Autodesk Fusion 360 part; units mm, degrees
sketch "Main Body" plane through (0, 0, 0) normal (0, 0, 1) x (1, 0, 0)
  circle A0 centre (0, 0) radius 16.85
  line L0 (-20, 20) -> (20, 20)
  line L1 (20, 20) -> (20, -20)
  line L2 (20, -20) -> (-20, -20)
  line L3 (-20, -20) -> (-20, 20)
  line L4 (-20, 15) -> (20, 15)
  point P0 (-20, 0)
  point P1 (0, 20)
  dimension "d1" = 33.7
  dimension "d2" = 40
  dimension "d3" = 15
extrude "Extrude1" add sketch "Main Body" along normal blind 30 contours A0 L1 L2 L3 L4
sketch "Antenna Holder" plane through (20, 0, 0) normal (1, 0, 0) x (0, 1, 0)
  line L0 (-20, 0) -> (15, 0)
  line L1 (15, 0) -> (15, 30)
  line L2 (15, 30) -> (-20, 30)
  line L3 (-20, 30) -> (-20, 0)
  circle A0 centre (-22.2, 9.1) radius 3.2
  line L4 (-23.48, 15) -> (-20, 15)
  line L5 (-20, 15) -> (-20, 0)
  line L6 (-20, 0) -> (-23.48, 0)
  line L7 (-23.48, 0) -> (-23.48, 15)
  point P0 (-23.48, 6.1672)
  dimension "d6" = 6.4
  dimension "d7" = 22.2
  dimension "d8" = 20.9
  dimension "d9" = 1.28
extrude "Extrude2" add sketch "Antenna Holder" against normal blind 40 contours L3 A0 L5 L6 L7 | L3 A0 L5 | L3 A0 L4 L5 L7
extrude "Extrude3" cut sketch "Antenna Holder" against normal blind 40 contours L3 A0 L5
sketch "Coax_Connector_holder" plane through (20, -21.74, 3.3881) normal (1, 0, 0) x (0, 1, 0)
  line L0 (-1.74, 2.779) -> (-13.74, 2.779)
  line L1 (-13.74, 2.779) -> (-13.74, -3.3881)
  line L2 (-13.74, -3.3881) -> (-1.74, -3.3881)
  line L3 (-1.74, -3.3881) -> (-1.74, 2.779)
  line L4 (1.74, -3.3881) -> (36.74, -3.3881)
  line L5 (-1.74, -3.3881) -> (-1.74, 11.6119)
  line L6 (-13.74, -3.3881) -> (-25.74, -3.3881)
  line L7 (-25.74, -3.3881) -> (-25.74, 11.6119)
  line L8 (-25.74, 11.6119) -> (-13.74, 11.6119)
  line L9 (-13.74, 11.6119) -> (-13.74, -3.3881)
  line L10 (-1.74, 11.6119) -> (1.74, 11.6119)
  point P0 (-1.74, 2.779)
  point P1 (-0.46, 5.7119)
  dimension "d15" = 12
  dimension "d16" = 12
extrude "Extrude4" add sketch "Coax_Connector_holder" against normal blind 40
sketch "Connector_Hole" plane through (0, -47.48, 0) normal (0, -1, 0) x (1, 0, 0)
  line L0 (20, 0) -> (20, 15)
  line L1 (20, 15) -> (-20, 15)
  line L2 (-20, 15) -> (-20, 0)
  line L3 (-20, 0) -> (20, 0)
  circle A0 centre (0, 11.1) radius 7.5
  circle A1 centre (0, 11.1) radius 8.5
  line L4 (-20, 30) -> (20, 30)
  line L5 (-20, 14.1) -> (20, 14.1)
  line L6 (-20, 14.5) -> (20, 14.5)
  dimension "d19" = 17
  dimension "d20" = 15
  dimension "d21" = 18.9
  dimension "d22" = 3
  dimension "d23" = 3.4
extrude "Extrude5" cut sketch "Connector_Hole" against normal blind 5.5 contours L0 A1 L5 L6 | L0 L1 A1 L6 | A0 A1 L5 L6 | L2 A1 L5 L6 | L1 A0 A1 L6 | A0 L5 L6 | A0 L5 | L1 L2 A1 L6 | A0 A1 L5 L6 | L1 A0 L6 | L1 A0 A1 L6
extrude "Extrude6" cut sketch "Connector_Hole" against normal blind 15 from surface at -5.5 contours L0 L1 A1 L6 | A0 A1 L5 L6 | A0 A1 L5 | L1 A0 A1 L6 | A0 L5 L6 | A0 L5 | L1 L2 A1 L6 | A0 A1 L5 L6 | L1 A0 L6 | L1 A0 A1 L6
sketch "Sketch5" plane through (0, 0, 15) normal (0, 0, 1) x (-1, 0, 0)
  line L0 (-20, 23.48) -> (-20, 20)
  line L1 (-20, 20) -> (20, 20)
  line L2 (20, 20) -> (20, 23.48)
  line L3 (20, 23.48) -> (-20, 23.48)
  line L4 (12, 20) -> (12, 23.48)
  line L5 (-12, 20) -> (-12, 23.48)
  dimension "d29" = 8
  dimension "d30" = 8
extrude "Extrude7" cut sketch "Sketch5" against normal blind 5 contours L1 L3 L4 L5
equation "d7 = 19 mm + 3.2 mm"
equation "d9 = d6 / 5"
equation "d10 = -d2"
equation "d12 = -d2"
equation "d17 = -d2"
equation "d21 = d8 - 2 mm"
equation "d22 = d20 / 5"
equation "d23 = d19 / 5"
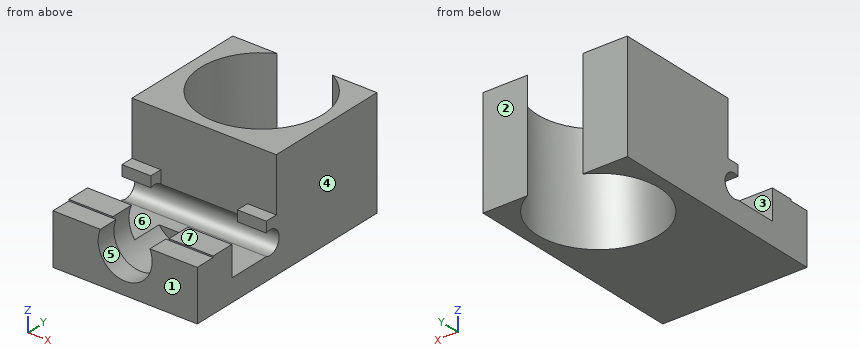
Input: part model. Units: mm. Frame: model coordinates. Face numbers are marked on the shaded views. A direction names the side the tool comes from. Give positions to 0.01 mm unless a question says otherwise; leave off trailing zeros. Order: outer loops, then holes, each group sorted by start corner. A loop starts at its lowest first (then second) coordinate and runs counter-clockwise, first axis right, second up. Notation, with made-up numbers: M 35.5,40 L 82.5,40 A25 cw 82.5,61 Z; hole C -31.5,19 d11. An arc over 180 degrees is marked long. Return JSON: item names as keys, results as strings.
Item 1: Cut plane A-A (y = -22.2). Return loops of the section in (x, z), then the cut area to 3 significant figures.
Solutions:
{"outline": "M -20,0 L 20,0 L 20,5.9 L -20,5.9 Z; M -20,12.3 L -12,12.3 L -12,15 L -20,15 Z; M 12,12.3 L 20,12.3 L 20,15 L 12,15 Z", "area": "279 mm^2"}
Item 2: Ray query, probe 1 along Y at (x, z) = (-9.5, 9); probe 2 along X at (y, z) = (-45.65, 11.1); probe 3 along X at (y, z) = (0, 9). Return the intervals inside material, ascending.
Solutions:
{"probe 1": "-47.48 to -35.48, -19 to -13.92, 13.92 to 15", "probe 2": "-20 to -7.5, 7.5 to 20", "probe 3": "-20 to -16.85, 16.85 to 20"}
Item 3: Pull-direction query (Y, two-part tool) for the marked faces 1, 2, 3 and 4; classes: +Y half, -Y half, draft (parallel to the pull), parting line (faces both ways), or undercut.
Solutions:
{"face 1": "-Y half", "face 2": "+Y half", "face 3": "undercut", "face 4": "draft"}
Item 4: Access query for the marked faces 5, 6 and 7. Directions: +Z, -Z, +X, -X, +Y, -Y. A direction counts if a zero-diameter tool reaches every point of the face in a straight line with its end or side. Return the directions, or none.
Solutions:
{"face 5": "-Y", "face 6": "+Z, +X, -X", "face 7": "+Z, +X, -X, -Y"}
Item 5: First-contact query: P1, Ø5, axis at x = -13.5, y = -37.5, coming from the +Z side; P2, Ø1.6, axis at x = -12.5, y = -43.5, coming from the +Z side; P3, Ø3, axis at x = -1, z = 7.5, coming from the +Y side. Flat tips, straight axial feed; report the tip coordinate or a pass-through.
Solutions:
{"P1": "z = 14.5", "P2": "z = 14.1", "P3": "y = -16.66"}
Item 6: Cut plane B-B (x = -10). Return loops of the section in (y, z).
Solutions:
{"outline": "M -47.48,0 L -13.56,0 L -13.56,30 L -20,30 L -20,11.42 A3.2 cw -23.48,6.17 L -35.48,6.17 L -35.48,14.5 L -41.98,14.5 L -41.98,14.1 L -47.48,14.1 Z; M 13.56,0 L 15,0 L 15,30 L 13.56,30 Z"}
Item 7: Cut plane C-C (z = 9.1). Return loops of the section in (x, y).
Solutions:
{"outline": "M -20,-47.48 L -7.23,-47.48 L -7.23,-41.98 L -8.26,-41.98 L -8.26,-35.48 L -20,-35.48 Z; M -20,-19 L 20,-19 L 20,15 L 7.68,15 A16.85 cw long -7.68,15 L -20,15 Z; M 7.23,-47.48 L 20,-47.48 L 20,-35.48 L 8.26,-35.48 L 8.26,-41.98 L 7.23,-41.98 Z"}
Item 8: Cut plane D-D (y = 0). Return loops of the section in (x, z).
Solutions:
{"outline": "M -20,0 L -16.85,0 L -16.85,30 L -20,30 Z; M 16.85,0 L 20,0 L 20,30 L 16.85,30 Z"}
